Part model, mm, in its own coordinate system. Face numbers are marked on the shaded views. Give positions to 0.01 mm unless a question says otherwise; leave off trailing zeros. Write each loop counter-clockwise with the first axis right and the second up, starting at its lowest first coordinate (ties: lowest second). Pieces come first, ordered by that corner, then holes. Notation, with made-up numbers: (27.25, 20.5) - (68.25, 20.5) arc R20 ccw to (68.25, 41.5) - close; hole circle Ø10 at (-28, 21.5). An arc over 180 degrees is marked (long way). Answer as a JSON object with one key per item and string values. Group by question number.
```python
from build123d import *

# Parameters (mm, degrees)
SKETCH2_W           = 71.12
SKETCH2_H           = 50.8
BOSS_EXTRUDE1_DEPTH = 12.7
FILLET2_R           = 6.35
SKETCH3_W           = 58.42
SKETCH3_H           = 39.37
CUT_EXTRUDE1_DEPTH  = 6.35
SKETCH4_W           = 3.81
SKETCH4_H           = 39.37
BOSS_EXTRUDE2_DEPTH = 4.318
LPATTERN1_COUNT     = 8
LPATTERN1_PITCH     = 7.62
SKETCH9_W           = 68.58
SKETCH9_H           = 12.7
CUT_EXTRUDE3_DEPTH  = 5.08
SKETCH10_R          = 2.54
BOSS_EXTRUDE3_DEPTH = 3.175
SKETCH8_W           = 30.144024865
SKETCH8_H           = 52.725935383
CUT_EXTRUDE2_DEPTH  = 83.82


with BuildPart() as part:
    # Sketch2 → Boss-Extrude1 (new body)
    with BuildSketch(Plane.XY):
        with Locations((35.56, 25.4)):
            Rectangle(SKETCH2_W, SKETCH2_H)
    extrude(amount=BOSS_EXTRUDE1_DEPTH)

    # Fillet2
    fillet2_edges = [part.edges().sort_by_distance(p)[0] for p in [
        (71.12, 25.4, 12.7),
        (35.56, 50.8, 12.7),
        (0, 25.4, 12.7),
    ]]
    fillet(fillet2_edges, radius=FILLET2_R)

    # Sketch3 → Cut-Extrude1 (cut)
    with BuildSketch(Plane.XY.offset(12.7)):
        with Locations((35.56, 24.765)):
            Rectangle(SKETCH3_W, SKETCH3_H)
    extrude(amount=-CUT_EXTRUDE1_DEPTH, mode=Mode.SUBTRACT)

    # Sketch4 → Boss-Extrude2 (add)
    with BuildSketch(Plane.XY.offset(6.35)):
        with Locations((8.255, 24.765)):
            Rectangle(SKETCH4_W, SKETCH4_H)
    boss_extrude2 = extrude(amount=BOSS_EXTRUDE2_DEPTH)

    # LPattern1: Boss-Extrude2 ×8
    with Locations(*[(i * LPATTERN1_PITCH, 0, 0) for i in range(1, LPATTERN1_COUNT)]):
        add(boss_extrude2)

    # Sketch7 → Revolve1 (revolve)
    with BuildSketch(Plane(origin=(6.35, 0, 0), x_dir=(0, 0, -1), z_dir=(1, 0, 0))):
        with BuildLine():
            Line((6.218866466, 44.45), (-15.24, 44.45))
            Line((-15.24, 44.45), (-15.24, 50.8))
            ThreePointArc((-15.24, 50.8), (-4.050658531, 49.179190459), (6.218866466, 44.45))
        make_face()
    revolve1 = revolve(axis=Axis((6.35, 44.45, -6.218866466), (0, 0, 1)))

    # Sketch9 → Cut-Extrude3 (cut)
    with BuildSketch(Plane(origin=(0, 0, 0), x_dir=(-1, 0, 0), z_dir=(0, 0, -1))):
        with Locations((-35.56, 9.525)):
            Rectangle(SKETCH9_W, SKETCH9_H)
    extrude(amount=-CUT_EXTRUDE3_DEPTH, mode=Mode.SUBTRACT)

    # Sketch10 → Boss-Extrude3 (add)
    with BuildSketch(Plane.ZY):
        with Locations((2.54, 25.4)):
            Circle(SKETCH10_R)
    boss_extrude3 = extrude(amount=BOSS_EXTRUDE3_DEPTH)

    # Mirror1: Revolve1, Boss-Extrude3 across plane
    add(revolve1.mirror(Plane(origin=(35.56, 0, 0), x_dir=(0, 0, 1), z_dir=(1, 0, 0))))
    add(boss_extrude3.mirror(Plane(origin=(35.56, 0, 0), x_dir=(0, 0, 1), z_dir=(1, 0, 0))))

    # Sketch8 → Cut-Extrude2 (cut)
    with BuildSketch(Plane.ZY):
        with Locations((-15.072012433, 24.437032309)):
            Rectangle(SKETCH8_W, SKETCH8_H)
    extrude(amount=-CUT_EXTRUDE2_DEPTH, mode=Mode.SUBTRACT)


solid = part.part
```
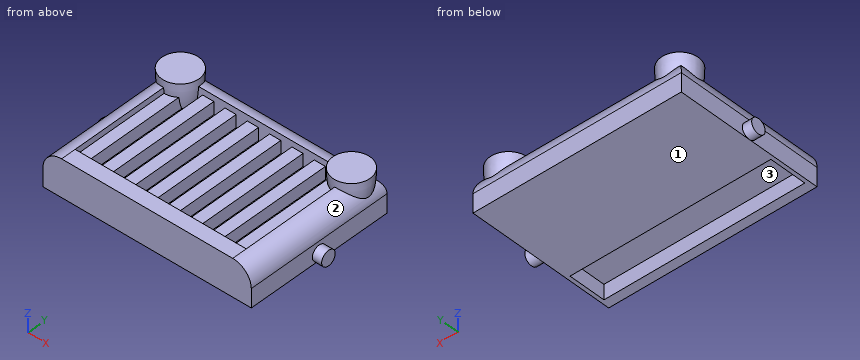
1) Probe line 1 (X direction, y = 10, z = 1); line 2 (Y direction, x = 42.5, z = 2) (3 decimals); line 3 (X direction, y = 17, z = 1). List the from-to ranges inside material, lowest first.
2) Mould opens along X. For the marked faces 1, 2 and 3 say: pulls with the +X half, pulls with the -X half, needs draft (parallel to the pull), parting line crosses it, or undercut.
3) Band-saw the part on A-A (z = 2.54). List the corners of the cut face in (x, y) (3 decimals).
4) Drop flat-ended pins along their axis: P1, Ø4, axis at x = 31.5, y = 28.5, coming from the +Z side; P2, Ø1, axis at y = 20.5, z = 12, coming from the +X side; P3, Ø8, axis at x = 15, y = 7.5, coming from the -Z side. Give the stop position or say it passes through.
5) Band-saw the part on B-B (x = 31). List the corners of the cut face in (y, z) (3 decimals), plus the area to 3 significant figures.
6) Band-saw the part on C-C (z = 9.75). State how many separate pieces and enclosed holes the cut face has, plus the area to 3 significant figures.
Verdict:
{
 "1": {"line 1": "0 to 1.27, 69.85 to 71.12", "line 2": "0 to 3.175, 15.875 to 50.8", "line 3": "0 to 71.12"},
 "2": {"face 1": "needs draft", "face 2": "pulls with the +X half", "face 3": "undercut"},
 "3": {"outline": "(-3.175, 22.86) - (0, 22.86) - (0, 0) - (71.12, 0) - (71.12, 22.86) - (74.295, 22.86) - (74.295, 27.94) - (71.12, 27.94) - (71.12, 50.8) - (0, 50.8) - (0, 27.94) - (-3.175, 27.94) - close; hole (1.27, 3.175) - (69.85, 3.175) - (69.85, 15.875) - (1.27, 15.875) - close"},
 "4": {"P1": "z = 10.67", "P2": "x = 68.48", "P3": "z = 5.08"},
 "5": {"outline": "(0, 0) - (3.175, 0) - (3.175, 5.08) - (15.875, 5.08) - (15.875, 0) - (50.8, 0) - (50.8, 6.35) arc R6.35 ccw to (44.45, 12.7) - (44.45, 10.668) - (5.08, 10.668) - (5.08, 12.7) - (0, 12.7) - close", "area": "492 mm2"},
 "6": {"separate pieces": "1", "enclosed holes": "8", "area": "2,370 mm2"}
}
